```python
from build123d import *

# Parameters (mm, degrees)
F1_DEPTH = 25.4
F2_DEPTH = 25.4


with BuildPart() as f1:
    # F0 (on Right) → F1 (new body)
    with BuildSketch(Plane.YZ):
        Polygon((-38.1, 0), (0, 0), (0, 12.7), (-25.4, 12.7), (-25.4, 31.75), (-38.1, 31.75), align=None)
    extrude(amount=F1_DEPTH)

    # F0 (on Right) → F2 (join)
    with BuildSketch(Plane.YZ):
        Polygon((-38.1, 0), (0, 0), (0, 12.7), (-25.4, 12.7), (-25.4, 31.75), (-38.1, 31.75), align=None)
    extrude(amount=F2_DEPTH)


solid = f1.part
```
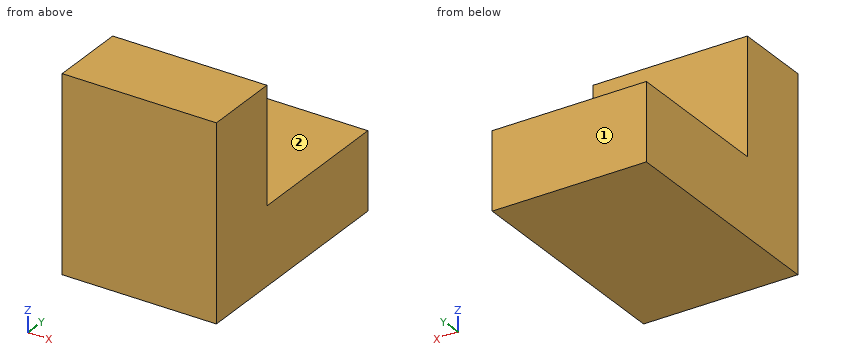
Can you work these out from the model? Positions are in its coordinate system, mm. Face numbers are marked on the shaded views. A direction names the side the tool comes from. Coordinates: 2 decimals unless noted, no trailing zeros. Loops run counter-clockwise (first coordinate to the right, second up) from the corner with the lowest first, then second, coordinate; pieces in that order, holes last.
1) Imagine slicing it at B-B on z = 16. List the corners of the cut face in (x, y) for me, plus the area to 3 significant figures.
2) Imagine slicing it at A-A on x = 9.25. List the corners of the cut face in (y, z) for me, plus the area to 3 significant figures.
3) Imagine slicing it at C-C on y = -11.5. List the corners of the cut face in (x, z) for me, plus the area to 3 significant figures.
4) Which directions (+Z, -Z, +X, -X, +Y, -Y) give clear straight access to the entire face, cutting with the end or side of a thin tool? Please do the marked faces 1 and 2.
5) I need wall thicknesses on probe 1 along Y at (x, z) = (13.5, 23.5); probe 2 along Z at (x, y) = (13.25, -5.5). Which ranges of each line are inside material? Lowest first, please.
6) For pin 1 (5 mm diameter, centred on x = 11, y = -18, fed in from +Z); pin 2 (1.5 mm diameter, centred on y = -23, z = 19, fed in from +X); pin 3 (8 mm diameter, centred on y = -33.5, z = 25.5, fed in from -X); pin 4 (9.5 mm diameter, centred on x = 14.5, z = 19, fed in from +Y), each with a flat end and sliding along its axis, tell me the tip position at first contact or that it passes through.
Completed:
1. outline: (0, -38.1) - (25.4, -38.1) - (25.4, -25.4) - (0, -25.4) - close
1. area: 323 mm2
2. outline: (-38.1, 0) - (0, 0) - (0, 12.7) - (-25.4, 12.7) - (-25.4, 31.75) - (-38.1, 31.75) - close
2. area: 726 mm2
3. outline: (0, 0) - (25.4, 0) - (25.4, 12.7) - (0, 12.7) - close
3. area: 323 mm2
4. face 1: +Z, -Z, +X, -X, +Y
4. face 2: +Z, +X, -X, +Y
5. probe 1: y = -38.1 to -25.4
5. probe 2: z = 0 to 12.7
6. pin 1: stops at z = 12.7
6. pin 2: passes through
6. pin 3: stops at x = 0
6. pin 4: stops at y = -25.4
